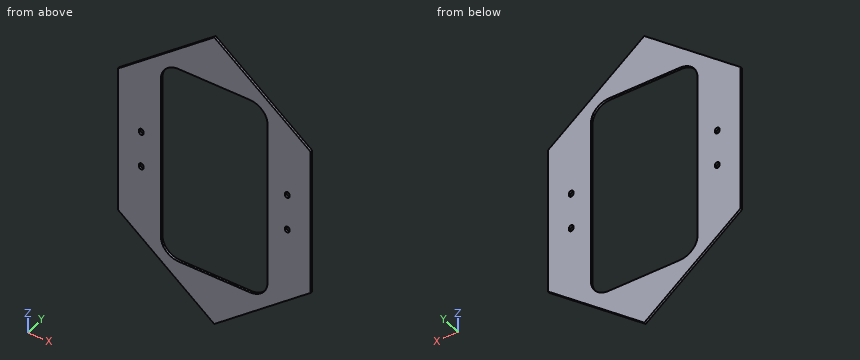
```python
from build123d import *

# Parameters (mm, degrees)
BOSS_EXTRUDE1_DEPTH = 3.175


with BuildPart() as part:
    # Sketch1 → Boss-Extrude1 (new body, symmetric)
    with BuildSketch(Plane(origin=(0, 0, 0), x_dir=(1, 0, 0), z_dir=(0, 1, 0))):
        Polygon((-276.225, 213.881843), (0, 434.861843), (276.225, 213.881843), (276.225, -213.881843), (0, -434.861843), (-276.225, -213.881843), align=None)
        with BuildLine():
            Line((101.6, -292.1), (-101.6, -292.1))
            ThreePointArc((-101.6, -292.1), (-137.521024484, -277.221024484), (-152.4, -241.3))
            Line((-152.4, -241.3), (-152.4, 241.3))
            ThreePointArc((-152.4, 241.3), (-137.521024484, 277.221024484), (-101.6, 292.1))
            Line((-101.6, 292.1), (101.6, 292.1))
            ThreePointArc((101.6, 292.1), (137.521024484, 277.221024484), (152.4, 241.3))
            Line((152.4, 241.3), (152.4, -241.3))
            ThreePointArc((152.4, -241.3), (137.521024484, -277.221024484), (101.6, -292.1))
        make_face(mode=Mode.SUBTRACT)
        with BuildLine():
            Line((-202.803125, 55.165625), (-202.803125, 49.609375))
            ThreePointArc((-202.803125, 49.609375), (-209.153125, 43.259375), (-215.503125, 49.609375))
            Line((-215.503125, 49.609375), (-215.503125, 55.165625))
            ThreePointArc((-215.503125, 55.165625), (-209.153125, 61.515625), (-202.803125, 55.165625))
        make_face(mode=Mode.SUBTRACT)
        with BuildLine():
            Line((-202.803125, -55.165625), (-202.803125, -49.609375))
            ThreePointArc((-202.803125, -49.609375), (-209.153125, -43.259375), (-215.503125, -49.609375))
            Line((-215.503125, -49.609375), (-215.503125, -55.165625))
            ThreePointArc((-215.503125, -55.165625), (-209.153125, -61.515625), (-202.803125, -55.165625))
        make_face(mode=Mode.SUBTRACT)
        with BuildLine():
            Line((202.803125, -55.165625), (202.803125, -49.609375))
            ThreePointArc((202.803125, -49.609375), (209.153125, -43.259375), (215.503125, -49.609375))
            Line((215.503125, -49.609375), (215.503125, -55.165625))
            ThreePointArc((215.503125, -55.165625), (209.153125, -61.515625), (202.803125, -55.165625))
        make_face(mode=Mode.SUBTRACT)
        with BuildLine():
            Line((202.803125, 55.165625), (202.803125, 49.609375))
            ThreePointArc((202.803125, 49.609375), (209.153125, 43.259375), (215.503125, 49.609375))
            Line((215.503125, 49.609375), (215.503125, 55.165625))
            ThreePointArc((215.503125, 55.165625), (209.153125, 61.515625), (202.803125, 55.165625))
        make_face(mode=Mode.SUBTRACT)
    extrude(amount=BOSS_EXTRUDE1_DEPTH, both=True)


solid = part.part
```
Here's how the part is built. I have some questions about the finished solid (model axes, mm). Give positions to 0.01 mm unless a question says otherwise; leave off trailing zeros. Loops run counter-clockwise (first coordinate to the right, second up) from the corner with the lowest first, then second, coordinate; pieces in that order, holes last. Notation, with made-up numbers: M 6,-31 L 24,-31 A27 ccw 24,-4 Z; hole C -36,72 d6. An arc over 180 degrees is marked long. Return JSON: item names as keys, results as strings.
Item 1: Imagine slicing it at A-A on y = -0.75. State how many separate pieces and enclosed holes the cut face has, then the cut area to 3 significant figures.
A:
{"separate pieces": "1", "enclosed holes": "5", "area": "182,000 mm^2"}
Item 2: I'm going to push flat-ended pins straight in: pin 1 Ø3 at (x, y) = (-62.5, 1) entering from -Z; pin 2 Ø1 at (x, y) = (73.5, -1.5) entering from +Z; pin 3 Ø1.9 at (x, y) = (-12.5, -1.5) entering from +Z. Where does each tip first touch, or does it pass through?
A:
{"pin 1": "stops at z = -386.06", "pin 2": "stops at z = 376.46", "pin 3": "stops at z = 425.62"}
Item 3: Imagine slicing it at C-C on x = 135. List the corners of the cut face in (y, z) for me (3 decimals), then the cut area to 3 significant figures.
A:
{"outline": "M -3.175,-326.862 L 3.175,-326.862 L 3.175,-279.576 L -3.175,-279.576 Z; M -3.175,279.576 L 3.175,279.576 L 3.175,326.862 L -3.175,326.862 Z", "area": "601 mm^2"}
Item 4: Imagine slicing it at B-B on z = -99.5. List the corners of the cut face in (x, y) for me (3 decimals).
A:
{"outline": "M -276.225,-3.175 L -152.4,-3.175 L -152.4,3.175 L -276.225,3.175 Z; M 152.4,-3.175 L 276.225,-3.175 L 276.225,3.175 L 152.4,3.175 Z"}
Item 5: Please list where these lines run through material, in increasing order: line 1 (X direction, y = -2.25, z = -132) (3 decimals); line 2 (X direction, y = -0.5, z = -47.5) (3 decimals); line 3 (Z direction, x = -203.5, y = 1.75).
A:
{"line 1": "x = -276.225 to -152.4, 152.4 to 276.225", "line 2": "x = -276.225 to -215.143, -203.164 to -152.4, 152.4 to 203.164, 215.143 to 276.225", "line 3": "z = -272.06 to -58.06, -46.72 to 46.72, 58.06 to 272.06"}
Item 6: Imagine slicing it at D-D on z = -326.5. List the corners of the cut face in (x, y) for me (3 decimals).
A:
{"outline": "M -135.452,-3.175 L 135.452,-3.175 L 135.452,3.175 L -135.452,3.175 Z"}
